CAD build for the part. Positions are in the model's coordinates, mm. A direction names the side the tool comes from. Give positions to 0.01 mm unless a question says otherwise; leave off trailing zeros. Loops run counter-clockwise (first coordinate to the right, second up) from the corner with the lowest first, then second, coordinate; pieces in that order, holes last. Notation, with made-up numbers: M -12.5,12.5 L 10.5,12.5 A17 ccw 10.5,28.5 Z; hole C -22,74 d2. An arc over 180 degrees is marked long. Answer as CSV lines item,"result".
from build123d import *

# Parameters (mm, degrees)
FILETE1_R                  = 2.5
FILETE2_R                  = 1.5
FILETE3_R                  = 2
FILETE4_R                  = 2
CORTE_EXTRUS_O2_DEPTH      = 10
CORTE_EXTRUS_O2_DEPTH_BACK = 10
ESBO_O3_OUTSIDE_W          = 44.606
ESBO_O3_OUTSIDE_H          = 44.606


with BuildPart() as part:
    # Esboço1 → Revolução1 (revolve)
    with BuildSketch(Plane.XY, mode=Mode.PRIVATE) as revolu_o1_sk:
        Polygon((8.1, -2.311461794), (8.1, -20.311461794), (5.35, -20.311461794), (5.35, -23.311461794), (10.75, -23.311461794), (10.75, -5.311461794), (16.25, -5.311461794), (16.25, -2.311461794), align=None)
    revolve(revolu_o1_sk.sketch.rotate(Axis((0, 66.826190476, 0), (0, -1, 0)), 90), axis=Axis((0, 66.826190476, 0), (0, -1, 0)))

    # Filete1
    filete1_edges = [part.edges().sort_by_distance(p)[0] for p in [
        (0, -2.311461794, -8.1),
    ]]
    fillet(filete1_edges, radius=FILETE1_R)

    # Filete2
    filete2_edges = [part.edges().sort_by_distance(p)[0] for p in [
        (0, -20.311461794, -8.1),
    ]]
    fillet(filete2_edges, radius=FILETE2_R)

    # Filete3
    filete3_edges = [part.edges().sort_by_distance(p)[0] for p in [
        (0, -23.311461794, -10.75),
    ]]
    fillet(filete3_edges, radius=FILETE3_R)

    # Filete4
    filete4_edges = [part.edges().sort_by_distance(p)[0] for p in [
        (0, -5.311461794, -10.75),
    ]]
    fillet(filete4_edges, radius=FILETE4_R)

    # Esboço3 outside → Corte-extrusão2 (cut, two sides: drawn at the far end of the back side and taken through both)
    with BuildSketch(Plane.XZ.offset(5.311461794).offset(-CORTE_EXTRUS_O2_DEPTH_BACK)):
        Rectangle(ESBO_O3_OUTSIDE_W, ESBO_O3_OUTSIDE_H)
        Polygon((-10.75, 0), (-10.75, -18.400139995), (10.75, -18.400139995), (10.75, 0), (10.75, 16.970186259), (-10.75, 16.970186259), align=None, mode=Mode.SUBTRACT)
    extrude(amount=CORTE_EXTRUS_O2_DEPTH + CORTE_EXTRUS_O2_DEPTH_BACK, mode=Mode.SUBTRACT)


solid = part.part
1) Band-saw the part on A-A on x = 0. Give the cut face in (y, z).
Answer below:
outline,"M -23.31,-8.75 A2 ccw -21.31,-10.75 L -7.31,-10.75 A2 cw -5.31,-12.75 L -5.31,-16.25 L -2.31,-16.25 L -2.31,-10.6 A2.5 ccw -4.81,-8.1 L -18.81,-8.1 A1.5 cw -20.31,-6.6 L -20.31,-5.35 L -23.31,-5.35 Z; M -23.31,5.35 L -20.31,5.35 L -20.31,6.6 A1.5 cw -18.81,8.1 L -4.81,8.1 A2.5 ccw -2.31,10.6 L -2.31,16.25 L -5.31,16.25 L -5.31,12.75 A2 cw -7.31,10.75 L -21.31,10.75 A2 ccw -23.31,8.75 Z"
2) Mould opens along X. For faces 1 (the face through (7.907, -11.909, -1.756)), 2 (the face through (-5.41, -20.311, -1.01)), 3 (the face through (-10.75, -4, 0)), 4 (the face through (0, -5.311, 14)) say: +X half, -X half, draft (parallel to the pull), parting line (faces both ways), or undercut.
Answer below:
face 1,"undercut"
face 2,"undercut"
face 3,"-X half"
face 4,"draft"
3) Drill centre lines: line 1 (X direction, y = -10, z = 0); line 2 (X direction, y = -21.45, z = 0); line 3 (Z direction, x = -5.5, y = -13.75). Where is each one in solid material? Low to high. Write a range as from..to.
Answer below:
line 1,"x = -10.75..-8.1, 8.1..10.75"
line 2,"x = -10.75..-5.35, 5.35..10.75"
line 3,"z = -9.24..-5.95, 5.95..9.24"
4) Flat gauge pins, fed straight in: pin 1 (6 mm diameter, centred on x = -2.5, y = -15, fed in from +Z); pin 2 (3 mm diameter, centred on y = -18, z = -2, fed in from +X); pin 3 (6 mm diameter, centred on y = -20, z = -11, fed in from -X). Where does each tip first touch, or does it go through?
Answer below:
pin 1,"stops at z = 10.75"
pin 2,"stops at x = 10.74"
pin 3,"stops at x = -7.18"
5) Band-saw the part on B-B on y = -16.25. Give the cut face in (x, z), and give its area (3 significant figures).
Answer below:
outline,"C 0,0 d21.5; hole C 0,0 d16.2"
area,"157 mm^2"
6) Which spindle directions (+Z, -Z, +X, -X, +Y, -Y) get a long thin tool onto all of the face, cutting with end or side? Do faces 5 (the face through (-0.16, -3.79, -16.25)), 6 (the face through (0, -5.311, -14)), 7 (the face through (-10.66, -14.21, -1.4)). Say none if no direction does.
Answer below:
face 5,"-Z, +Y, -Y"
face 6,"-Z, -Y"
face 7,"-Y"
